Can you work these out from the model? Positions are in its coordinate system, mm. Give positions to 0.01 mm unless a question says otherwise; leave off trailing zeros. Order: outer loops, then holes, each group sorted by start corner. A loop starts at its lowest first (then second) coordinate and runs counter-clockwise, first axis right, second up. Notation, with made-up numbers: M 13,67.5 L 58,67.5 A27 ccw 58,96.5 Z; hole C 71,57 d3. An arc over 180 degrees is marked long. Answer as a JSON object with one key per item and string values.
```python
from build123d import *

# Parameters (mm, degrees)
SKETCH1_W           = 393.7
SKETCH1_H           = 63.5
BOSS_EXTRUDE1_DEPTH = 6.35
SKETCH2_R           = 3.3655
SKETCH2_R_2         = 2.5527
CUT_EXTRUDE1_DEPTH  = 200.49513152


with BuildPart() as part:
    # Sketch1 → Boss-Extrude1 (new body)
    with BuildSketch(Plane(origin=(0, 0, 0), x_dir=(1, 0, 0), z_dir=(0, 1, 0))):
        Rectangle(SKETCH1_W, SKETCH1_H)
    extrude(amount=BOSS_EXTRUDE1_DEPTH)

    # Sketch2 → Cut-Extrude1 (cut, through all)
    with BuildSketch(Plane.XZ):
        with Locations(Location((-92.062267829, 0, 0), (0, 0, 270))):
            Circle(SKETCH2_R)
        with Locations((-92.062267829, 0)):
            Circle(SKETCH2_R_2, mode=Mode.SUBTRACT)
        with Locations((-92.062267829, 0)):
            Circle(SKETCH2_R_2)
        with Locations(Location((-184.15, 6.35, 0), (0, 0, 270))):
            Circle(SKETCH2_R)
        with Locations(Location((-184.15, -19.05, 0), (0, 0, 270))):
            Circle(SKETCH2_R)
        with Locations(Location((92.075, 0, 0), (0, 0, 270))):
            Circle(SKETCH2_R)
        with Locations((92.075, 0)):
            Circle(SKETCH2_R_2, mode=Mode.SUBTRACT)
        with Locations((92.075, 0)):
            Circle(SKETCH2_R_2)
        with Locations(Location((184.15, 6.35, 0), (0, 0, 270))):
            Circle(SKETCH2_R)
        with Locations(Location((184.15, -19.05, 0), (0, 0, 270))):
            Circle(SKETCH2_R)
    extrude(amount=-CUT_EXTRUDE1_DEPTH, mode=Mode.SUBTRACT)


solid = part.part
```
1) Thinking about a two-plate mould opening in Z: for faces 1 (the face through (-180.813, 3.131, -18.612)), 2 (the face through (-196.85, 3, 0)), 3 (the face through (-3, 3, 31.75)), which applies, pulls with the +Z half, pulls with the -Z half, needs draft (parallel to the pull), parting line crosses it, or undercut?
Results found:
{"face 1": "undercut", "face 2": "needs draft", "face 3": "pulls with the +Z half"}
2) I want a section at B-B on z = -19.05. Write out the boundary of the cut face in (x, y).
Results found:
{"outline": "M -196.85,0 L -187.52,0 L -187.52,6.35 L -196.85,6.35 Z; M -180.78,0 L 180.78,0 L 180.78,6.35 L -180.78,6.35 Z; M 187.52,0 L 196.85,0 L 196.85,6.35 L 187.52,6.35 Z"}
3) I want a section at A-A on x = 184.15. Write out the boundary of the cut face in (y, z), and give its area (3 significant figures).
Results found:
{"outline": "M 0,-31.75 L 6.35,-31.75 L 6.35,-22.42 L 0,-22.42 Z; M 0,-15.68 L 6.35,-15.68 L 6.35,2.98 L 0,2.98 Z; M 0,9.72 L 6.35,9.72 L 6.35,31.75 L 0,31.75 Z", "area": "318 mm²"}
4) I need wall thicknesses on L1, parallel to Z at x = -184.15, y = 2; L2, parallel to X at y = 2, z = -0.5; L3, parallel to X at y = 5.25, z = 6.35. Which ranges of each line are inside material? Lowest first, please.
Results found:
{"L1": "z = -31.75 to -22.42, -15.68 to 2.98, 9.72 to 31.75", "L2": "x = -196.85 to -95.39, -88.73 to 88.75, 95.4 to 196.85", "L3": "x = -196.85 to -187.52, -180.78 to 180.78, 187.52 to 196.85"}
